Model file for the job. Use its own axes, mm. A direction names the side the tool comes from. Give positions to 0.01 mm unless a question says otherwise; leave off trailing zeros. Loops run counter-clockwise (first coordinate to the right, second up) from the corner with the lowest first, then second, coordinate; pieces in that order, holes last. Notation, with made-up numbers: (-14.5, 28.5) - (30.5, 28.5) arc R24 ccw to (30.5, 51.5) - close; hole circle Ø4 at (-37, -37). An arc over 180 degrees is marked (long way). Use a Markdown table: item, result.
from build123d import *

# Parameters (mm, degrees)
SKETCH1_W           = 20
SKETCH1_H           = 15
BOSS_EXTRUDE2_DEPTH = 2
BOSS_EXTRUDE3_DEPTH = 3


with BuildPart() as part:
    # Sketch1 → Boss-Extrude2 (new body)
    with BuildSketch(Plane.XY):
        with Locations((10, 7.5)):
            Rectangle(SKETCH1_W, SKETCH1_H)
    extrude(amount=BOSS_EXTRUDE2_DEPTH)

    # Sketch2 → Boss-Extrude3 (add)
    with BuildSketch(Plane.XY.offset(2)):
        Polygon((1, 15), (0, 15), (0, 14), (0, 12), (1, 12), (1, 14), (3, 14), (3, 15), align=None)
        Polygon((1, 3), (0, 3), (0, 1), (0, 0), (1, 0), (3, 0), (3, 1), (1, 1), align=None)
        Polygon((19, 15), (17, 15), (17, 14), (19, 14), (19, 12), (20, 12), (20, 14), (20, 15), align=None)
        Polygon((20, 0), (17, 0), (17, 1), (19, 1), (19, 3), (20, 3), align=None)
    extrude(amount=BOSS_EXTRUDE3_DEPTH)


solid = part.part
(1) Slice it at D-D, the plane x = 10.5. Write the cut outline in (y, z).
Computed:
| item | result |
|---|---|
| outline | (0, 0) - (15, 0) - (15, 2) - (0, 2) - close |
(2) Slice it at B-B, the plane y = 12.25. Write the cut outline in (x, z).
Computed:
| item | result |
|---|---|
| outline | (0, 0) - (20, 0) - (20, 5) - (19, 5) - (19, 2) - (1, 2) - (1, 5) - (0, 5) - close |
(3) Slice it at A-A, the plane z = 4.2. Write the cut outline in (x, y), plus the area to 3 significant figures.
Computed:
| item | result |
|---|---|
| outline | (0, 0) - (3, 0) - (3, 1) - (1, 1) - (1, 3) - (0, 3) - close; (0, 12) - (1, 12) - (1, 14) - (3, 14) - (3, 15) - (0, 15) - close; (17, 0) - (20, 0) - (20, 3) - (19, 3) - (19, 1) - (17, 1) - close; (17, 14) - (19, 14) - (19, 12) - (20, 12) - (20, 15) - (17, 15) - close |
| area | 20.0 mm² |
(4) 3-axis set-ups, long thin cutter, end or side, ignore diameter. For faces 4 (the flat face through (2, 1, 3)), 5 (the flat face through (17, 14.5, 3.5)), 6 (the flat face through (19.5, 3, 3.5)): which of +Z, -Z, +X, -X, +Y, -Y reach the whole face in a straight line?
Computed:
| item | result |
|---|---|
| face 4 | +Z |
| face 5 | +Z, +Y, -Y |
| face 6 | +Z, +X, -X |
(5) Slice it at C-C, the plane x = 2. Write the cut outline in (y, z), plus the area to 3 significant figures.
Computed:
| item | result |
|---|---|
| outline | (0, 0) - (15, 0) - (15, 5) - (14, 5) - (14, 2) - (1, 2) - (1, 5) - (0, 5) - close |
| area | 36.0 mm² |
(6) Mould opens along X. For faces 1 (the flat face through (19, 2, 3)), 2 (the flat face through (0, 8, 1)), 3 (the flat face through (0.5, 3, 3.5)) say: pulls with the +X half, pulls with the -X half, needs draft (parallel to the pull), parting line crosses it, or undercut.
Computed:
| item | result |
|---|---|
| face 1 | undercut |
| face 2 | pulls with the -X half |
| face 3 | needs draft |
(7) Pin check, flat tip, straight feed: P1, Ø6, axis at x = 6.5, y = 6, coming from the +Z side. Stop position of the tip, or through.
Computed:
| item | result |
|---|---|
| P1 | z = 2 |
(8) Drill centre lines: probe 1 along Y at (x, z) = (1.5, 2.8); probe 2 along Z at (x, y) = (10.5, 4.5); probe 3 along X at (y, z) = (1.25, 4.05). Where is each one in solid material? Low to high. Write a range as [from, to].
Computed:
| item | result |
|---|---|
| probe 1 | [0, 1], [14, 15] |
| probe 2 | [0, 2] |
| probe 3 | [0, 1], [19, 20] |
